from build123d import *

# Parameters (mm, degrees)
CYLINDER001_R          = 1.625
CYLINDER001_DEPTH      = 10
CYLINDER001_ROLL_ANGLE = -90
PAD_DEPTH              = 1.25
CYLINDER_R             = 8.5
CYLINDER_DEPTH         = 10
SKETCH001_R            = 2.625
POCKET_DEPTH           = 1.5
POCKET001_DEPTH        = 6.5
SKETCH004_W            = 18
SKETCH004_H            = 2
POCKET002_DEPTH        = 10.001
CHAMFER_SIZE           = 2
SKETCH005_R            = 10
POCKET003_DEPTH        = 3
POLARPATTERN_COUNT     = 5
CHAMFER001_SIZE        = 1


with BuildPart() as wheelrevolution:
    # Sketch → Revolution (revolve)
    with BuildSketch(Plane.XZ):
        Polygon((34.5, 5), (36.5, 3), (36.5, 2.12132), (34.37868, 0), (36.5, -2.12132), (36.5, -3), (32.5, -3), (27.5, 2), (0, 2), (0, 5), align=None)
    revolve(axis=Axis((0, 0, 0), (0, 0, 1)))


with BuildPart() as wheelshaftscrewcylinder001:
    # Cylinder001 → Cylinder001 (new body)
    with BuildSketch(Plane.XY):
        Circle(CYLINDER001_R)
    extrude(amount=CYLINDER001_DEPTH)


with BuildPart() as wheelshaftscrewcylinder001_1:
    # Cylinder001 roll: moved
    add(wheelshaftscrewcylinder001.part.rotate(Axis((0, 0, 0), (1, 0, 0)), CYLINDER001_ROLL_ANGLE))


with BuildPart() as wheelshaftscrewcylinder001_2:
    # Cylinder001 placement: moved
    add(wheelshaftscrewcylinder001_1.part.moved(Location((0, 0, -2))))


with BuildPart() as wheelshaftnutscrewfusion:
    # Sketch003 → Pad (new body, symmetric)
    with BuildSketch(Plane.XZ):
        Polygon((2.875, -5), (2.875, 1.659882), (0, 3.319764), (-2.875, 1.659882), (-2.875, -5), align=None)
    extrude(amount=PAD_DEPTH, both=True)


with BuildPart() as wheelshaftnutscrewfusion_1:
    # Clone placement: moved
    add(wheelshaftnutscrewfusion.part.moved(Location((0, 4.875, -2))))

    # Fusion: union WheelShaftScrewCylinder001
    add(wheelshaftscrewcylinder001_2.part)


with BuildPart() as wheelcutoutchamfer001_final:
    # Cylinder → Cylinder (new body)
    with BuildSketch(Plane.XY.offset(-6)):
        Circle(CYLINDER_R)
    extrude(amount=CYLINDER_DEPTH)

    # Sketch001 → Pocket (cut)
    with BuildSketch(Plane(origin=(0, 0, -6), x_dir=(1, 0, 0), z_dir=(0, 0, -1))):
        Circle(SKETCH001_R)
    extrude(amount=-POCKET_DEPTH, mode=Mode.SUBTRACT)

    # Sketch002 → Pocket001 (cut)
    with BuildSketch(Plane(origin=(0, 0, -4.5), x_dir=(1, 0, 0), z_dir=(0, 0, -1))):
        with BuildLine():
            ThreePointArc((-2.061553, 1.625), (0, -2.625), (2.061553, 1.625))
            Line((2.061553, 1.625), (-2.061553, 1.625))
        make_face()
    extrude(amount=-POCKET001_DEPTH, mode=Mode.SUBTRACT)

    # Cut: cut WheelShaftNutScrewFusion
    add(wheelshaftnutscrewfusion_1.part, mode=Mode.SUBTRACT)

    # Sketch004 → Pocket002 (cut, through all)
    with BuildSketch(Plane(origin=(0, 0, -6), x_dir=(1, 0, 0), z_dir=(0, 0, -1))):
        with Locations((0, -8.625)):
            Rectangle(SKETCH004_W, SKETCH004_H)
    extrude(amount=-POCKET002_DEPTH, mode=Mode.SUBTRACT)

    # Fusion001: union WheelRevolution
    add(wheelrevolution.part)

    # Chamfer
    chamfer_edges = [wheelcutoutchamfer001_final.edges().sort_by_distance(p)[0] for p in [
        (-4.490096, -7.217274, 2),
    ]]
    chamfer(chamfer_edges, length=CHAMFER_SIZE)

    # Sketch005 → Pocket003 (cut, symmetric)
    with BuildSketch(Plane(origin=(0, 0, 2), x_dir=(1, 0, 0), z_dir=(0, 0, -1))):
        with Locations((0, 20)):
            Circle(SKETCH005_R)
    pocket003 = extrude(amount=POCKET003_DEPTH, both=True, mode=Mode.SUBTRACT)

    # PolarPattern: Pocket003 ×5 about axis
    polarpattern_axis = Axis((0, 0, 2), (0, 0, -1))
    for i in range(1, POLARPATTERN_COUNT):
        add(pocket003.rotate(polarpattern_axis, i * 360 / POLARPATTERN_COUNT), mode=Mode.SUBTRACT)

    # Chamfer001
    chamfer001_edges = [wheelcutoutchamfer001_final.edges().sort_by_distance(p)[0] for p in [
        (19.845875, 10.302487, 5),
        (15.93096, -15.690905, 5),
        (-10, -20, 5),
        (-22.1113, 3.330225, 5),
        (-3.665535, 22.058192, 5),
    ]]
    chamfer(chamfer001_edges, length=CHAMFER001_SIZE)


solid = wheelcutoutchamfer001_final.part
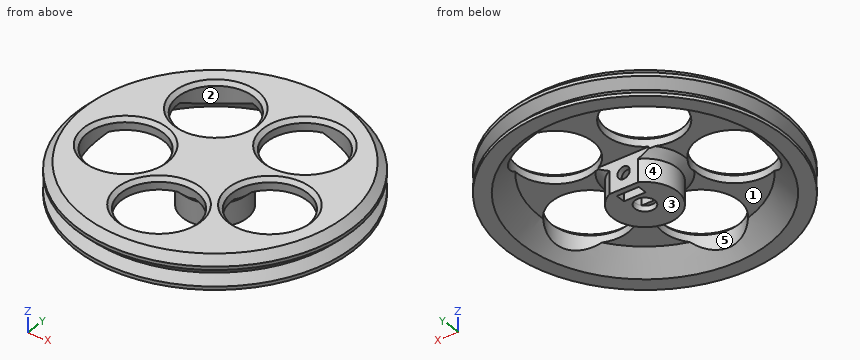
For this review, take the finished solid that the model builds, in its own axes (mm). Face numbers are marked on the shaded views. A direction names the side the tool comes from. Coordinates: 2 decimals unless noted, no trailing zeros. Use a Markdown table: item, result. Add a question column.
Item 1: We need section A-A (x = 17). Give the number of separate pieces and of enclosed holes in the cut face, and give its area (3 significant figures).
Item 2: Insertion check: pin 1 Ø4 at (y, z) = (-7.5, 0) entering from -X; pin 2 Ø1.5 at (y, z) = (19.5, 2.5) entering from +X; pin 3 Ø4.5 at (x, z) = (0, -2.5) entering from +Y. Each pin has a flat end and moves straight along its axis. Give the tip position at first contact, or say it passes through.
Item 3: Mouldability with a two-part tool opening along X and no side actions: class the marked faces 1, 2 and 3 as pulls with the +X half, pulls with the -X half, needs draft (parallel to the pull), parting line crosses it, or undercut.
Item 4: For line 1 (X direction, y = -9.5, z = 4.25); line 2 (Y direction, x = -15, z = 3.75); line 3 (X direction, y = 1.5, z = -1), list the stretches that pass through material, from the lowest coordinate up.
Item 5: Tool access review of the marked faces 4 and 5: name each direction out of +Z, -Z, +X, -X, +Y, -Y from which nothing blocks a thin tool from reaching the whole face with its end or side.
Results list:
| question | item | result |
|---|---|---|
| 1 | separate pieces | 3 |
| 1 | enclosed holes | 0 |
| 1 | area | 139 mm^2 |
| 2 | pin 1 | stops at x = -35.64 |
| 2 | pin 2 | stops at x = 31.32 |
| 2 | pin 3 | stops at y = 36.5 |
| 3 | face 1 | undercut |
| 3 | face 2 | undercut |
| 3 | face 3 | needs draft |
| 4 | line 1 | x = -33.95 to -28.72, -9.32 to 9.32, 28.72 to 33.95 |
| 4 | line 2 | y = -32.45 to -15.34, 2.98 to 6.72, 25.64 to 32.45 |
| 4 | line 3 | x = -35.35 to -30.46, -8.37 to -2.15, 2.15 to 8.37, 30.46 to 35.35 |
| 5 | face 4 | -Z |
| 5 | face 5 | +Z, -Z |
